Answer from the drawing. Dimensions are ordinates in mm from the lowest x, y and z of the part. Coordinates: 2 decimals unless noted, no trailing zeros. Write each loop counter-clockwise with the first axis right and the second up, starting at its lowest first coordinate (ties: lowest second). Pieces come first, ordered by that corner, then holes. Notation, with made-up numbers: (29, -19) - (80, -19) arc R19 ccw to (80, -9) - close; hole circle Ø8 at (78, 84). An arc over 180 degrees is marked (long way). Answer as a JSON object with one key per item and string values. Group by question number.
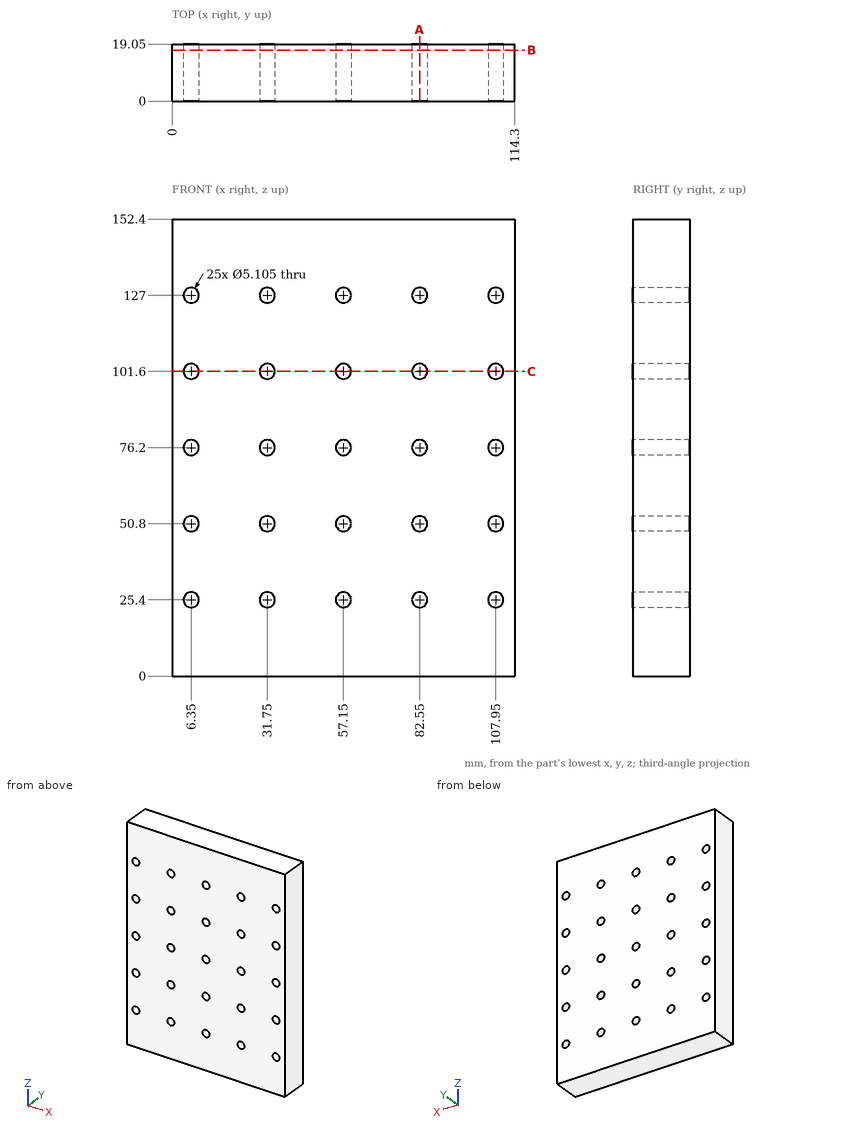
Q1. Section C-C on z = 101.6 is taken. Determine the outline of the cut face in (x, y).
Q2. Section A-A on x = 82.55 is taken. Determine the outline of the cut face in (y, z), plus the area to 3 significant figures.
Q3. Consider L1, parallel to Z at x = 108, y = 4.75; L2, parallel to X at y = 9, z = 101.6; L3, parallel to Z at x = 56.5, y = 15.75. Determine where each line is inside the solid, lowest interval first. Write a range as from..to.
Q4. Section B-B on y = 17 is taken. Count the separate pieces of the cut face and the enclosed holes in it, plus the area to 3 significant figures.
Numbers:
{
 "1": {"outline": "(0, 0) - (3.8, 0) - (3.8, 19.05) - (0, 19.05) - close; (8.9, 0) - (29.2, 0) - (29.2, 19.05) - (8.9, 19.05) - close; (34.3, 0) - (54.6, 0) - (54.6, 19.05) - (34.3, 19.05) - close; (59.7, 0) - (80, 0) - (80, 19.05) - (59.7, 19.05) - close; (85.1, 0) - (105.4, 0) - (105.4, 19.05) - (85.1, 19.05) - close; (110.5, 0) - (114.3, 0) - (114.3, 19.05) - (110.5, 19.05) - close"},
 "2": {"outline": "(0, 0) - (19.05, 0) - (19.05, 22.85) - (0, 22.85) - close; (0, 27.95) - (19.05, 27.95) - (19.05, 48.25) - (0, 48.25) - close; (0, 53.35) - (19.05, 53.35) - (19.05, 73.65) - (0, 73.65) - close; (0, 78.75) - (19.05, 78.75) - (19.05, 99.05) - (0, 99.05) - close; (0, 104.15) - (19.05, 104.15) - (19.05, 124.45) - (0, 124.45) - close; (0, 129.55) - (19.05, 129.55) - (19.05, 152.4) - (0, 152.4) - close", "area": "2,420 mm²"},
 "3": {"L1": "z = 0..22.85, 27.95..48.25, 53.35..73.65, 78.75..99.05, 104.15..124.45, 129.55..152.4", "L2": "x = 0..3.8, 8.9..29.2, 34.3..54.6, 59.7..80, 85.1..105.4, 110.5..114.3", "L3": "z = 0..22.93, 27.87..48.33, 53.27..73.73, 78.67..99.13, 104.07..124.53, 129.47..152.4"},
 "4": {"separate pieces": "1", "enclosed holes": "25", "area": "16,900 mm²"}
}
